from build123d import *

# Parameters (mm, degrees)
OTHER_START         = 7.189240539
OTHER_2_OUTLINE_W   = 16
OTHER_2_OUTLINE_H   = 16
OTHER_2_DEPTH       = 1.9877561
SKETCH_20_R         = 2.8
EXTRUDE_2_DEPTH     = 6.5
SKETCH_22_R         = 4
CUT_EXTRUDE_2_DEPTH = 9
CUT_EXTRUDE_3_DEPTH = 0.5


# Read off the part's stored shape, not the designer's step: 相交2
with BuildPart() as part:
    # 草图4 → Loft 1 section 0
    with BuildSketch(Plane(origin=(0, 8.2, 0), x_dir=(1, 0, 0), z_dir=(0, 1, 0))):
        with BuildLine():
            Line((-5.6, 6.8), (5.6, 6.8))
            Line((5.6, 6.8), (5.6, -5.7))
            Line((5.6, -5.7), (-5.6, -5.7))
            Line((-5.6, -5.7), (-5.6, 6.8))
        make_face()
    # 草图1 → Loft 1 section 1
    with BuildSketch(Plane(origin=(0, 0, 0), x_dir=(1, 0, 0), z_dir=(0, 1, 0))):
        with BuildLine():
            Line((-8.95, -8.9), (8.95, -8.9))
            Line((8.95, -8.9), (8.95, 8.9))
            Line((8.95, 8.9), (-8.95, 8.9))
            Line((-8.95, 8.9), (-8.95, -8.9))
        make_face()
    loft()

    # 相交2 outline → 相交2 (cut)
    with BuildSketch(Plane(origin=(0, 0, 0), x_dir=(1, 0, 0), z_dir=(0, 0.9872752829851917, -0.15902048800865198)).offset(OTHER_START)):
        Rectangle(OTHER_2_OUTLINE_W, OTHER_2_OUTLINE_H)
    extrude(amount=OTHER_2_DEPTH, mode=Mode.SUBTRACT)

    # 草图19 → Loft 1 2 section 0
    with BuildSketch(Plane(origin=(0, 6.132664073, -0.987788564), x_dir=(1, 0, 0), z_dir=(0, 0.9872752829851916, -0.15902048800865207))):
        with BuildLine():
            Line((-4.985089723, 5.299749211), (4.985089723, 5.299749211))
            Line((4.985089723, 5.299749211), (4.287230721, -5.442213697))
            Line((4.287230721, -5.442213697), (-4.287230721, -5.442213697))
            Line((-4.287230721, -5.442213697), (-4.985089723, 5.299749211))
        make_face()
    # 草图8 → Loft 1 2 section 1
    with BuildSketch(Plane.XZ):
        with BuildLine():
            Line((-7.15, 7.2), (7.15, 7.2))
            Line((7.15, 7.2), (7.15, -7.5))
            Line((7.15, -7.5), (-7.15, -7.5))
            Line((-7.15, -7.5), (-7.15, 7.2))
        make_face()
    loft(mode=Mode.SUBTRACT)

    # 草图20 → 凸台-拉伸2 (add)
    with BuildSketch(Plane.XZ):
        with Locations(Location((0, 0, 0), (0, 0, 270))):
            Circle(SKETCH_20_R)
        Polygon((-2.2, 0.8), (-0.8, 0.8), (-0.8, 2.2), (0.8, 2.2), (0.8, 0.8), (2.2, 0.8), (2.2, -0.8), (0.8, -0.8), (0.8, -2.2), (-0.8, -2.2), (-0.8, -0.8), (-2.2, -0.8), align=None, mode=Mode.SUBTRACT)
    extrude(amount=-EXTRUDE_2_DEPTH)

    # 草图22 → 切除-拉伸2 (cut)
    with BuildSketch(Plane.XZ):
        with Locations((7, 9)):
            Circle(SKETCH_22_R)
    extrude(amount=-CUT_EXTRUDE_2_DEPTH, mode=Mode.SUBTRACT)

    # 草图23 → 切除-拉伸3 (cut)
    with BuildSketch(Plane(origin=(0, 7.097759487, -1.143236539), x_dir=(1, 0, 0), z_dir=(0, 0.9872752829851916, -0.15902048800865207))):
        with BuildLine():
            Line((-0.979801877, 3.777052641), (-1.249032646, 3.521844308))
            add(Edge.make_bspline(
                [(-1.249032646, 3.521844308), (-1.297751534, 3.567675171), (-1.39402758, 3.658244034), (-1.550987823, 3.775755029), (-1.714751457, 3.876421129), (-1.884463954, 3.958327366), (-2.055922508, 4.023680126), (-2.226851284, 4.070208266), (-2.395496985, 4.099880804), (-2.507664204, 4.103429173), (-2.562934889, 4.105177641)],
                knots=[0, 0, 0, 0, 1.08915593, 2.152340314, 3.188132944, 4.216796309, 5.218260357, 6.173443236, 7.099959455, 8, 8, 8, 8], degree=3))
            add(Edge.make_bspline(
                [(-2.562934889, 4.105177641), (-2.596849589, 4.104764035), (-2.66459103, 4.103937896), (-2.765212974, 4.093393681), (-2.864779611, 4.078228817), (-2.963102986, 4.056286939), (-3.060374272, 4.02847788), (-3.156255164, 3.993692417), (-3.250924519, 3.953137172), (-3.3434906, 3.906274699), (-3.433231104, 3.854794852), (-3.517987939, 3.797746312), (-3.598301338, 3.736957522), (-3.672661763, 3.670906542), (-3.74149695, 3.600191677), (-3.806445322, 3.526128371), (-3.865222618, 3.446693152), (-3.918313783, 3.363347526), (-3.965675401, 3.277555337), (-4.007484055, 3.190142347), (-4.042581143, 3.101398493), (-4.070350598, 3.011212415), (-4.093261252, 2.920281825), (-4.109378859, 2.827977105), (-4.118465582, 2.73419942), (-4.120037361, 2.671402161), (-4.120827518, 2.63983309)],
                knots=[0, 0, 0, 0, 1.02818874, 2.053710826, 3.065248034, 4.081641283, 5.106893873, 6.131558223, 7.173050175, 8.228653731, 9.27666206, 10.308777013, 11.325269123, 12.329503258, 13.32196095, 14.316845687, 15.314881793, 16.315733098, 17.311955233, 18.285320748, 19.252783886, 20.203351036, 21.145449891, 22.095197417, 23.042428769, 24, 24, 24, 24], degree=3))
            add(Edge.make_bspline(
                [(-4.120827518, 2.63983309), (-4.120071799, 2.607562273), (-4.118562426, 2.543108759), (-4.108902107, 2.446914687), (-4.090973866, 2.352149284), (-4.067006157, 2.258501151), (-4.037025342, 2.165809903), (-3.999652676, 2.074477393), (-3.955387075, 1.984507002), (-3.904150523, 1.896709385), (-3.84796432, 1.811186362), (-3.785021239, 1.73062684), (-3.718160655, 1.653958063), (-3.644946755, 1.582882299), (-3.567727213, 1.515498403), (-3.484194937, 1.453662881), (-3.395992477, 1.396184658), (-3.302985265, 1.343788138), (-3.206182482, 1.296979603), (-3.106925729, 1.255355706), (-3.004897914, 1.221076369), (-2.900635224, 1.193138265), (-2.794261952, 1.170237968), (-2.68523815, 1.155505488), (-2.574365441, 1.144814657), (-2.499626809, 1.144032987), (-2.461973351, 1.14363918)],
                knots=[0, 0, 0, 0, 0.93586088, 1.869166235, 2.799637598, 3.729985548, 4.670839027, 5.622275134, 6.589130586, 7.576015415, 8.568469353, 9.55398029, 10.53834874, 11.515998671, 12.510579167, 13.508179873, 14.527009472, 15.561807829, 16.601455013, 17.643573243, 18.680854198, 19.719860599, 20.772568776, 21.833555941, 22.908541556, 24, 24, 24, 24], degree=3))
            add(Edge.make_bspline(
                [(-2.461973351, 1.14363918), (-2.416595004, 1.144587756), (-2.327487246, 1.14645044), (-2.196500804, 1.160950729), (-2.070697733, 1.183597523), (-1.95043153, 1.21676342), (-1.835562509, 1.259067095), (-1.725669568, 1.310062481), (-1.621617909, 1.37170554), (-1.523094735, 1.441279407), (-1.43233755, 1.51879424), (-1.350483426, 1.602438695), (-1.278837937, 1.691806762), (-1.216333237, 1.786372077), (-1.164624583, 1.886917382), (-1.122181788, 1.992949944), (-1.089648496, 2.104517456), (-1.076293522, 2.181609088), (-1.069545466, 2.220562257)],
                knots=[0, 0, 0, 0, 1.13008108, 2.219097802, 3.278683437, 4.311054135, 5.322181354, 6.324827112, 7.324222904, 8.330512327, 9.32562643, 10.293043162, 11.24128371, 12.174520618, 13.111833804, 14.052305215, 15.015860969, 16, 16, 16, 16], degree=3))
            Line((-1.069545466, 2.220562257), (-2.236212133, 2.220562257))
            Line((-2.236212133, 2.220562257), (-2.236212133, 2.579536616))
            Line((-2.236212133, 2.579536616), (-0.755442902, 2.579536616))
            add(Edge.make_bspline(
                [(-0.755442902, 2.579536616), (-0.757148751, 2.512629127), (-0.760487404, 2.381679085), (-0.78390632, 2.190708814), (-0.821722832, 2.010337121), (-0.873383144, 1.840374049), (-0.940258424, 1.681060457), (-1.021630952, 1.53223459), (-1.118803074, 1.39485791), (-1.228313515, 1.267808906), (-1.351213473, 1.154479694), (-1.484182093, 1.054873756), (-1.627439061, 0.970971141), (-1.780848869, 0.902710478), (-1.943909302, 0.849436483), (-2.116997682, 0.811664907), (-2.299879283, 0.789034943), (-2.425215959, 0.786143564), (-2.489317101, 0.784664821)],
                knots=[0, 0, 0, 0, 1.140356446, 2.231883559, 3.274166699, 4.278491846, 5.25512956, 6.21435461, 7.1637429, 8.11826594, 9.068280886, 10.0076534, 10.945064095, 11.891975133, 12.864533718, 13.863980011, 14.907571808, 16, 16, 16, 16], degree=3))
            add(Edge.make_bspline(
                [(-2.489317101, 0.784664821), (-2.528827236, 0.785233942), (-2.606753957, 0.786356433), (-2.721844885, 0.79433378), (-2.833762506, 0.806614356), (-2.942490515, 0.82515948), (-3.048428857, 0.847874134), (-3.151048442, 0.876960853), (-3.250740184, 0.910629552), (-3.347658169, 0.948925226), (-3.440922716, 0.993296882), (-3.530949233, 1.042606522), (-3.618235359, 1.096599882), (-3.702186524, 1.156210728), (-3.783240145, 1.220993188), (-3.860873589, 1.291077107), (-3.935521467, 1.366248227), (-3.982281931, 1.419627237), (-4.005843543, 1.446523795)],
                knots=[0, 0, 0, 0, 1.107784379, 2.184907829, 3.233506516, 4.263428166, 5.276301166, 6.270063455, 7.25232949, 8.225834625, 9.190232166, 10.146266622, 11.1027726, 12.066435141, 13.031522626, 14.010570082, 14.99756817, 16, 16, 16, 16], degree=3))
            add(Edge.make_bspline(
                [(-4.005843543, 1.446523795), (-4.040029475, 1.489194448), (-4.107833888, 1.573827465), (-4.195112044, 1.70942741), (-4.269513447, 1.84982927), (-4.329881269, 1.995423898), (-4.377019356, 2.146075111), (-4.410825608, 2.301590402), (-4.430632898, 2.462170033), (-4.433486435, 2.570835298), (-4.434930082, 2.625810654)],
                knots=[0, 0, 0, 0, 1.023165419, 2.029347347, 3.013907458, 3.994755782, 4.975994455, 5.96558838, 6.970761222, 8, 8, 8, 8], degree=3))
            add(Edge.make_bspline(
                [(-4.434930082, 2.625810654), (-4.434397844, 2.666976907), (-4.433340132, 2.748786214), (-4.420514615, 2.870243522), (-4.402113197, 2.989544214), (-4.375066143, 3.10659077), (-4.340969878, 3.221461362), (-4.298416392, 3.334209326), (-4.248871496, 3.444901197), (-4.191286, 3.552775065), (-4.127201541, 3.656399478), (-4.05765132, 3.755357282), (-3.98164772, 3.847846347), (-3.90043192, 3.935037995), (-3.81303493, 4.015836842), (-3.720275507, 4.090990953), (-3.622082164, 4.160601138), (-3.518145984, 4.223570973), (-3.410018299, 4.280134594), (-3.297958298, 4.329723805), (-3.182000187, 4.370707121), (-3.063012709, 4.4054809), (-2.940095209, 4.431196041), (-2.814139672, 4.449844786), (-2.68448956, 4.462605386), (-2.59685353, 4.463631642), (-2.552418062, 4.464152)],
                knots=[0, 0, 0, 0, 1.008945113, 2.00506715, 2.99143336, 3.967273523, 4.948097931, 5.927297278, 6.919902385, 7.919676788, 8.923139349, 9.905703106, 10.883022732, 11.856032218, 12.825136022, 13.798837087, 14.781400844, 15.773989409, 16.776158564, 17.77167057, 18.775803737, 19.789618931, 20.80898985, 21.851988756, 22.910860228, 24, 24, 24, 24], degree=3))
            add(Edge.make_bspline(
                [(-2.552418062, 4.464152), (-2.516179819, 4.463572509), (-2.44432364, 4.462423445), (-2.337397908, 4.454458797), (-2.232124893, 4.441834915), (-2.128348503, 4.424608129), (-2.026422137, 4.401144438), (-1.926055432, 4.373066154), (-1.827102895, 4.340374331), (-1.729874646, 4.301385485), (-1.63371693, 4.25713186), (-1.53809509, 4.207318437), (-1.443335844, 4.151093433), (-1.349274862, 4.088289897), (-1.255319004, 4.019986479), (-1.162954362, 3.944229656), (-1.069951418, 3.8640069), (-1.010149603, 3.806324716), (-0.979801877, 3.777052641)],
                knots=[0, 0, 0, 0, 0.985871117, 1.954866573, 2.915460327, 3.869826059, 4.81536089, 5.759505086, 6.70452669, 7.649098992, 8.607881297, 9.583363685, 10.581137262, 11.603961102, 12.659522466, 13.73993555, 14.853081303, 16, 16, 16, 16], degree=3))
        make_face()
    extrude(amount=-CUT_EXTRUDE_3_DEPTH, mode=Mode.SUBTRACT)


solid = part.part
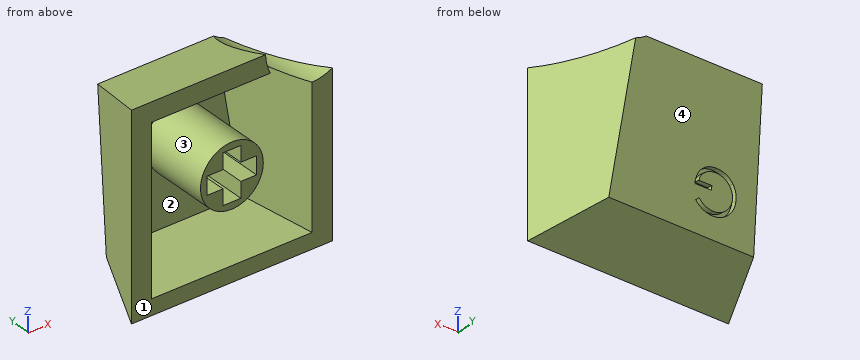
Could you check a few things on this model? Use its own coordinates, in mm. Face numbers are marked on the shaded views. Round coordinates to 2 decimals unless told otherwise and drop trailing zeros.
Q1. Thinking about a two-plate mould opening in Z: for the marked faces 1, 2, 3 and 4, which applies, released by +Z, released by -Z, zero draft, split by the parting line, or undercut?
Geometry says:
face 1: zero draft
face 2: undercut
face 3: undercut
face 4: released by -Z
Q2. Imagine slicing it at A-A, the plane y = 4.75. State how many separate pieces and enclosed holes the cut face has, then the cut area to 3 significant figures.
Geometry says:
separate pieces: 2
enclosed holes: 2
area: 93.3 mm2
Q3. I'm going to push flat-ended pins straight in: P1, Ø1.3, axis at x = 0, y = 3, coming from the +Z side; P2, Ø0.5, axis at y = 3.5, z = 0.5, coming from the +X side; P3, Ø0.5, axis at x = 0.5, z = 2.5, coming from the +Y side; P4, Ø5, axis at x = -5.5, z = 1.5, coming from the -Y side. Where does each tip first touch, or does it pass through?
Geometry says:
P1: stops at z = 7.98
P2: stops at x = 7.62
P3: stops at y = 7.72
P4: stops at y = 0
Q4. Please list where these lines run through material, in increasing order: probe 1 along Z at (x, y) = (0, 3.25); probe 2 along Z at (x, y) = (1, 4.5); probe 3 along X at (y, z) = (5.25, -0.25).
Geometry says:
probe 1: z = -8.07 to -6.71, -2.8 to -2.2, 2.2 to 2.8, 5.89 to 7.63
probe 2: z = -7.75 to -6.41, -2.62 to -0.8, 0.8 to 2.62, 5.39 to 7.14
probe 3: x = -6.81 to -5, -2.79 to -2.2, 2.2 to 2.79, 5 to 6.81
